Check sheet for the drawn part. Datum: minimum x, y, z corner. Units: mm. A direction names the side the tool comes from. Round coordinates to 2 decimals unless told otherwise and drop trailing zeros. Order: outer loops, then holes, each group sorted by start corner. A loop starts at its lowest first (then second) coordinate and runs counter-clockwise, first axis right, second up.
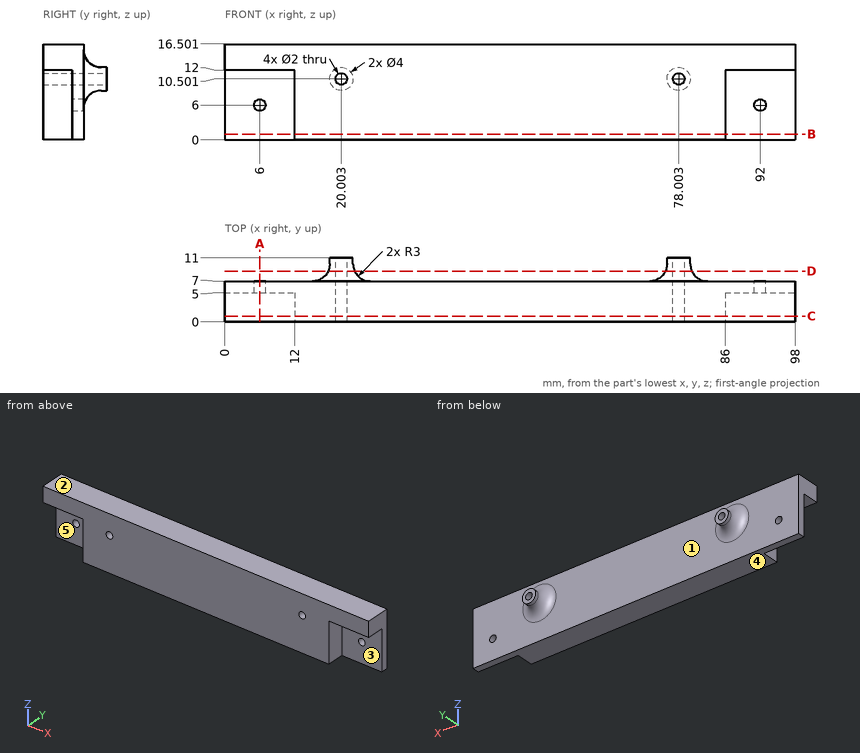
1) Gauge pin test, flat ends, axial feed: pin 1 (2.5 mm diameter, centred on x = 92, z = 6, fed in from +Y); pin 2 (2.5 mm diameter, centred on x = 92, y = 2, fed in from -Z); pin 3 (1.5 mm diameter, centred on y = 3.5, z = 8.5, fed in from -X). Record the tip position at first contact, or that the pin passes through.
2) Draft check along X on the marked faces 1 and 2. Enter one of: pulls with the +X half, pulls with the -X half, needs draft (parallel to the pull), parting line crosses it, or undercut.
3) Set-up check for the marked faces 3, 4 and 5: record each of +Z, -Z, +X, -X, +Y, -Y from which the full face is reachable in a straight line by a thin tool's end or side.
4) Sectioned sample at B-B on z = 1. Record the cut outline in (x, y), and give its area (3 significant figures).
5) Scan lines: line 1 (X direction, y = 6.45, z = 6); line 2 (X direction, y = 0.5, z = 10.5); line 3 (X direction, y = 3.25, z = 1.25). Record each from-to range of solid material in increasing order.
6) Sectioned sample at A-A on x = 6. Record the cut outline in (y, z), and give its area (3 significant figures).
7) Sectioned sample at C-C on y = 1. Record the cut outline in (x, z).
8) Sectioned sample at D-D on y = 8.75. Record the cut outline in (x, z) (1 decimal).
Values found:
1. pin 1: stops at y = 7
1. pin 2: stops at z = 12
1. pin 3: stops at x = 12
2. face 1: undercut
2. face 2: needs draft
3. face 3: -Z, +X, -Y
3. face 4: -Z, +X, -X, +Y, -Y
3. face 5: -Z, -X, -Y
4. outline: (0, 5) - (12, 5) - (12, 0) - (86, 0) - (86, 5) - (98, 5) - (98, 7) - (0, 7) - close
4. area: 566 mm2
5. line 1: x = 0 to 5, 7 to 91, 93 to 98
5. line 2: x = 12 to 19, 21 to 77, 79 to 86
5. line 3: x = 12 to 86
6. outline: (0, 12) - (5, 12) - (5, 7) - (7, 7) - (7, 16.5) - (0, 16.5) - close; (5, 0) - (7, 0) - (7, 5) - (5, 5) - close
6. area: 51.5 mm2
7. outline: (0, 12) - (12, 12) - (12, 0) - (86, 0) - (86, 12) - (98, 12) - (98, 16.5) - (0, 16.5) - close; hole circle Ø2 at (20, 10.5); hole circle Ø2 at (78, 10.5)
8. outline: circle Ø4.5 at (20, 10.5); circle Ø4.5 at (78, 10.5); hole circle Ø2 at (20, 10.5); hole circle Ø2 at (78, 10.5)
